```python
from build123d import *

# Parameters (mm, degrees)
F0_R     = 8.905875
F1_DEPTH = 9.525
F2_R     = 12.954
F2_R_2   = 8.905875
F3_DEPTH = 34.29


with BuildPart() as f1:
    # F0 (on Front) → F1 (new body)
    with BuildSketch(Plane.XZ):
        Polygon((-48.517683, 30.776316), (-53.640253, 28.657804), (-53.45877, 31.42681), (-58.260996, 28.657804), (-58.442479, 31.42681), (-62.842216, 28.054681), (-63.383566, 30.776316), (-67.305504, 26.858747), (-68.197476, 29.486428), (-71.574508, 25.090476), (-72.801836, 27.579244), (-75.576176, 22.780092), (-77.117854, 25.087377), (-79.242056, 19.967169), (-81.071695, 22.053499), (-82.509411, 16.699814), (-84.595716, 18.529478), (-85.322334, 13.033934), (-87.629619, 14.575612), (-87.632718, 9.032265), (-90.121486, 10.259593), (-89.40099, 4.763262), (-92.02867, 5.655234), (-90.596923, 0.299974), (-93.318559, 0.84135), (-91.200046, -4.281246), (-93.969053, -4.099738), (-91.200046, -8.901963), (-93.969053, -9.083472), (-90.596923, -13.483184), (-93.318559, -14.024534), (-89.40099, -17.946472), (-92.02867, -18.838443), (-87.632718, -22.215475), (-90.121486, -23.442803), (-85.322334, -26.217143), (-87.629619, -27.758822), (-82.509411, -29.883024), (-84.595716, -31.712687), (-79.242056, -33.150378), (-81.071695, -35.236709), (-75.576176, -35.963301), (-77.117854, -38.270586), (-71.574508, -38.273685), (-72.801836, -40.762453), (-67.305504, -40.041957), (-68.197476, -42.669638), (-62.842216, -41.237891), (-63.383566, -43.959526), (-58.260996, -41.841014), (-58.442479, -44.61002), (-53.640253, -41.841014), (-53.45877, -44.61002), (-49.059059, -41.237891), (-48.517683, -43.959526), (-44.595771, -40.041957), (-43.703799, -42.669638), (-40.326767, -38.273685), (-39.099439, -40.762453), (-36.325073, -35.963301), (-34.783395, -38.270586), (-32.659218, -33.150378), (-30.829555, -35.236709), (-29.391864, -29.883024), (-27.305533, -31.712687), (-26.578916, -26.217143), (-24.27163, -27.758822), (-24.268557, -22.215475), (-21.779789, -23.442803), (-22.500285, -17.946472), (-19.872604, -18.838443), (-21.304352, -13.483184), (-18.582716, -14.024534), (-20.701203, -8.901963), (-17.932197, -9.083472), (-20.701203, -4.281246), (-17.932197, -4.099738), (-21.304352, 0.299974), (-18.582716, 0.84135), (-22.500285, 4.763262), (-19.872604, 5.655234), (-24.268557, 9.032265), (-21.779789, 10.259593), (-26.578916, 13.033934), (-24.27163, 14.575612), (-29.391864, 16.699814), (-27.305533, 18.529478), (-32.659218, 19.967169), (-30.829555, 22.053499), (-36.325073, 22.780092), (-34.783395, 25.087377), (-40.326767, 25.090476), (-39.099439, 27.579244), (-44.595771, 26.858747), (-43.703799, 29.486428), (-49.059059, 28.054681), align=None)
        with Locations((-55.950637, -6.591605)):
            Circle(F0_R, mode=Mode.SUBTRACT)
    extrude(amount=F1_DEPTH)

    # F2 (on face) → F3 (cut)
    with BuildSketch(Plane.XZ.offset(9.525)):
        with Locations((-55.950637, -6.591605)):
            Circle(F2_R)
        with Locations((-55.950637, -6.591605)):
            Circle(F2_R_2, mode=Mode.SUBTRACT)
    extrude(amount=-F3_DEPTH, mode=Mode.SUBTRACT)


solid = f1.part
```
For this review, take the finished solid that the model builds, in its own axes (mm). Round coordinates to 2 decimals unless told otherwise and drop trailing zeros. Order: outer loops, then holes, each group sorted by start corner. A loop starts at its lowest first (then second) coordinate and runs counter-clockwise, first axis right, second up.
Q1. We need section A-A, the plane z = 2. Give the boundary of the cut face in (x, y) (1 decimal), plus the area to 3 significant figures.
Findings below:
outline: (-91.1, -9.5) - (-65.6, -9.5) - (-65.6, 0) - (-91.1, 0) - close; (-46.3, -9.5) - (-19.7, -9.5) - (-19.7, 0) - (-46.3, 0) - close
area: 495 mm2
Q2. We need section B-B, the plane x = -46. Give the boundary of the cut face in (y, z) (3 decimals).
Findings below:
outline: (-9.525, -41.445) - (0, -41.445) - (0, -14.886) - (-9.525, -14.886) - close; (-9.525, 1.702) - (0, 1.702) - (0, 28.873) - (-9.525, 28.873) - close
Q3. Mouldability with a two-part tool opening along Z and no side actions: class faces 1 (the flat face through (-51.29, -4.7, -42.95)), 2 (the flat face through (-78.165, -4.696, 22.563)), 3 (the flat face through (-91.323, -4.696, 3.015)) as pulls with the +Z half, pulls with the -Z half, needs draft (parallel to the pull), parting line crosses it, or undercut.
Findings below:
face 1: pulls with the -Z half
face 2: pulls with the +Z half
face 3: undercut
Q4. Insertion check: P1, Ø1, axis at y = -2.5, z = -29, coming from the +X side; P2, Ø3, axis at y = -1, z = -4.5, coming from the -X side; P3, Ø4, axis at y = -7.5, z = 4.5, coming from the +X side; P4, Ø1.5, axis at x = -35, y = -1.5, coming from the -Z side. Each pin has a flat end and moves straight along its axis. Give the tip position at first contact, or say it passes through.
Findings below:
P1: stops at x = -26.88
P2: stops at x = -93.97
P3: stops at x = -19.87
P4: stops at z = -38.27
Q5. Wall thickness on line 1 (Z direction, x = -88, y = -8); line 2 (Z direction, x = -39.5, y = -4.25); line 3 (X direction, y = -4.25, z = 17): over which ranges is each line inside the solid? List them lowest first.
Findings below:
line 1: z = -24.67 to -22.4, -21.93 to 9.21
line 2: z = -39.95 to 25.09, 26.77 to 27.53
line 3: x = -84.8 to -82.85, -82.43 to -29.05
